from build123d import *

# Parameters (mm, degrees)
F0_R     = 3.175
F1_DEPTH = 6.35
F2_W     = 6.35
F2_H     = 24.715454
F2_H_2   = 28.652428
F3_DEPTH = 50.8
F4_R     = 2.54


with BuildPart() as f1:
    # F0 (on Right) → F1 (new body, symmetric)
    with BuildSketch(Plane.YZ):
        with BuildLine():
            Line((-22.225, -12.7), (0, -12.7))
            ThreePointArc((0, -12.7), (12.7, 0), (0, 12.7))
            Line((0, 12.7), (-22.225, 12.7))
            ThreePointArc((-22.225, 12.7), (-34.925, 0), (-22.225, -12.7))
        make_face()
        with Locations((-22.225, 0)):
            Circle(F0_R, mode=Mode.SUBTRACT)
        Circle(F0_R, mode=Mode.SUBTRACT)
    extrude(amount=F1_DEPTH, both=True)

    # F2 (on Front) → F3 (cut, symmetric)
    with BuildSketch(Plane.XZ):
        with Locations((0, 21.882727)):
            Rectangle(F2_W, F2_H)
        with Locations((0, -23.851214)):
            Rectangle(F2_W, F2_H_2)
    extrude(amount=F3_DEPTH, both=True, mode=Mode.SUBTRACT)

    # F4
    f4_edges = [f1.edges().sort_by_distance(p)[0] for p in [
        (-3.175, -11.1125, 9.525),
        (3.175, -11.1125, 9.525),
        (-3.175, -11.1125, -9.525),
        (3.175, -11.1125, -9.525),
    ]]
    fillet(f4_edges, radius=F4_R)


solid = f1.part
Could you check a few things on this model? Use its own coordinates, in mm. A direction names the side the tool comes from. Give positions to 0.01 mm unless a question says otherwise; leave off trailing zeros. Order: outer loops, then holes, each group sorted by start corner. A loop starts at its lowest first (then second) coordinate and runs counter-clockwise, first axis right, second up.
1. We'd pull the mould along Y, two halves only. Please class faces 1 (the cylindrical face through (0.09, -34.92, 0.28)), 2 (the cylindrical face through (-0.089, -19.197, 0.954)), 3 (the flat face through (0, -11, 9.525)): pulls with the +Y half, pulls with the -Y half, needs draft (parallel to the pull), parting line crosses it, or undercut.
2. Suppose I cut it at A-A (z = 0). List the corners of the cut face in (x, y) for me (3 decimals).
3. Will these pins go through, and if not, where does the flat tip stop? P1, Ø5, axis at x = 3, z = 8.5, coming from the +Y side; P2, Ø5, axis at x = 4.5, z = -8, coming from the +Y side; P3, Ø1, axis at x = 0.5, y = -11.5, coming from the -Z side; P4, Ø5.5, axis at y = -22.225, z = 0, coming from the +X side.
4. Suppose I cut it at B-B (x = 0). List the corners of the cut face in (y, z) for me (3 decimals), plus the area to 3 significant figures.
5. Suppose I cut it at C-C (z = -11). List the corners of the cut face in (x, y) for me.
6. For faces 4 (the flat face through (5, -11, 12.7)), 5 (the cylindrical face through (2.45, -10.84, -10.29)), 6 (the cylindrical face through (-2.45, -11.39, 10.29)), which set-ups out of +Z, -Z, +X, -X, +Y, -Y let a thin tool reach every point of the face, with its end or its side?
7. Suppose I cut it at D-D (z = 4). List the corners of the cut face in (x, y) for me.
8. I need wall thicknesses on L1, parallel to Z at x = 0.75, y = 0 (3 decimals); L2, parallel to Z at x = -3.75, y = 4; L3, parallel to X at y = -29, z = 10. Which ranges of each line are inside material? Lowest first, please.
Solved:
1. face 1: pulls with the -Y half
1. face 2: undercut
1. face 3: needs draft
2. outline: (-6.35, -34.925) - (6.35, -34.925) - (6.35, -25.4) - (-6.35, -25.4) - close; (-6.35, -19.05) - (6.35, -19.05) - (6.35, -3.175) - (-6.35, -3.175) - close; (-6.35, 3.175) - (6.35, 3.175) - (6.35, 12.7) - (-6.35, 12.7) - close
3. P1: stops at y = 11.19
3. P2: stops at y = 11.45
3. P3: stops at z = -9.55
3. P4: passes through
4. outline: (-30.625, -9.525) - (8.4, -9.525) arc R12.7 ccw to (8.4, 9.525) - (-30.625, 9.525) arc R12.7 ccw to start; hole circle Ø6.35 at (-22.225, 0); hole circle Ø6.35 at (0, 0)
4. area: 794 mm2
5. outline: (-6.35, -28.57) - (-2.94, -28.57) - (-2.94, 6.35) - (-6.35, 6.35) - close; (2.94, -28.57) - (6.35, -28.57) - (6.35, 6.35) - (2.94, 6.35) - close
6. face 4: +Z, +X, -X, +Y, -Y
6. face 5: -Z, +Y, -Y
6. face 6: +Z, +Y, -Y
7. outline: (-6.35, -34.28) - (6.35, -34.28) - (6.35, 12.05) - (-6.35, 12.05) - close
8. L1: z = -9.528 to -3.175, 3.175 to 9.528
8. L2: z = -12.05 to 12.05
8. L3: x = -6.35 to -2.11, 2.11 to 6.35
